from build123d import *


with BuildPart() as part:
    # Sketch1 → Revolve1 (revolve)
    with BuildSketch(Plane.XY):
        Polygon((12.7, 9.525), (15.875, 9.525), (15.875, 8.763), (22.225, 8.763), (22.225, 9.525), (25.4, 9.525), (25.4, 0), (12.7, 0), align=None)
    revolve(axis=Axis((0, 0, 0), (0, 1, 0)))

    # Mirror1: part across plane


with BuildPart() as part_1:
    add(part.part)
    add(part.part.mirror(Plane.ZX))


solid = part_1.part
Input: part model. Units: mm. Frame: model coordinates. A direction names the side the tool comes from. Coordinates: 2 decimals unless noted, no trailing zeros. Order: outer loops, then holes, each group sorted by start corner. A loop starts at its lowest first (then second) coordinate and runs counter-clockwise, first axis right, second up. Notation, with made-up numbers: M 27,14 L 72,14 A31 ccw 72,42 Z; hole C -24.5,21.5 d8. An arc over 180 degrees is marked long. Write item = value, one per line. Start each with the question number.
(1) Line query: line 1 along X through (y, z) = (-9.1, 0) (3 decimals); line 2 along Z through (x, y) = (0, -3.75). Output: solid intervals per line, ascending. Write a range as [from, to].
(2) Section B-B on x = 0. Output: boundary loops of the cut face in (y, z) (3 decimals).
(3) Section D-D on x = 19. Output: boundary loops of the cut face in (y, z) (3 decimals), and give its area (3 significant figures).
(4) Section A-A on z = 0. Output: boundary loops of the cut face in (x, y) (3 decimals).
(5) Pull-direction query (X, two-part tool) for faces 1 (the flat face through (-10, -8.763, 15)), 2 (the flat face through (0.1, -9.525, 22.5)); classes: released by +X, released by -X, zero draft, split by the parting line, or undercut.
(6) Reachability of faces 3 (the flat face through (0.1, 9.525, 22.5)), 4 (the cylindrical face through (-3.441, -9.139, 15.497)), 5 (the cylindrical face through (21.199, 9.149, -6.676)) from +Z, -Z, +X, -X, +Y, -Y: full face, straight path, thin tool, end or side. Return the list, or none.
(7) Section C-C on y = -3. Output: boundary loops of the cut face in (x, z).
(8) First-contact query: P1, Ø4, axis at y = -3.5, z = -12, coming from the +X side; P2, Ø5, axis at y = 3, z = -14, coming from the -X side; P3, Ø1, axis at y = -2.5, z = 20.5, coming from the -X side; P4, Ø8, axis at x = 13.5, z = -14.5, coming from the +Y side (3 decimals). Flat tips, straight axial feed; report the tip coordinate or a pass-through.
Result set:
q1.line_1 = [-25.4, -22.225], [-15.875, -12.7], [12.7, 15.875], [22.225, 25.4]
q1.line_2 = [-25.4, -12.7], [12.7, 25.4]
q2.outline = M -9.525,-25.4 L 9.525,-25.4 L 9.525,-22.225 L 8.763,-22.225 L 8.763,-15.875 L 9.525,-15.875 L 9.525,-12.7 L -9.525,-12.7 L -9.525,-15.875 L -8.763,-15.875 L -8.763,-22.225 L -9.525,-22.225 Z; M -9.525,12.7 L 9.525,12.7 L 9.525,15.875 L 8.763,15.875 L 8.763,22.225 L 9.525,22.225 L 9.525,25.4 L -9.525,25.4 L -9.525,22.225 L -8.763,22.225 L -8.763,15.875 L -9.525,15.875 Z
q3.outline = M -9.525,-16.857 L 9.525,-16.857 L 9.525,-11.53 L 8.763,-11.53 L 8.763,11.53 L 9.525,11.53 L 9.525,16.857 L -9.525,16.857 L -9.525,11.53 L -8.763,11.53 L -8.763,-11.53 L -9.525,-11.53 Z
q3.area = 607 mm²
q4.outline = M -25.4,-9.525 L -22.225,-9.525 L -22.225,-8.763 L -15.875,-8.763 L -15.875,-9.525 L -12.7,-9.525 L -12.7,9.525 L -15.875,9.525 L -15.875,8.763 L -22.225,8.763 L -22.225,9.525 L -25.4,9.525 Z; M 12.7,-9.525 L 15.875,-9.525 L 15.875,-8.763 L 22.225,-8.763 L 22.225,-9.525 L 25.4,-9.525 L 25.4,9.525 L 22.225,9.525 L 22.225,8.763 L 15.875,8.763 L 15.875,9.525 L 12.7,9.525 Z
q5.face_1 = undercut
q5.face_2 = zero draft
q6.face_3 = +Z, -Z, +X, -X, +Y
q6.face_4 = -Y
q6.face_5 = +Y
q7.outline = C 0,0 d50.8; hole C 0,0 d25.4
q8.P1 = 23.35
q8.P2 = -22.65
q8.P3 = -15.66
q8.P4 = 9.525
